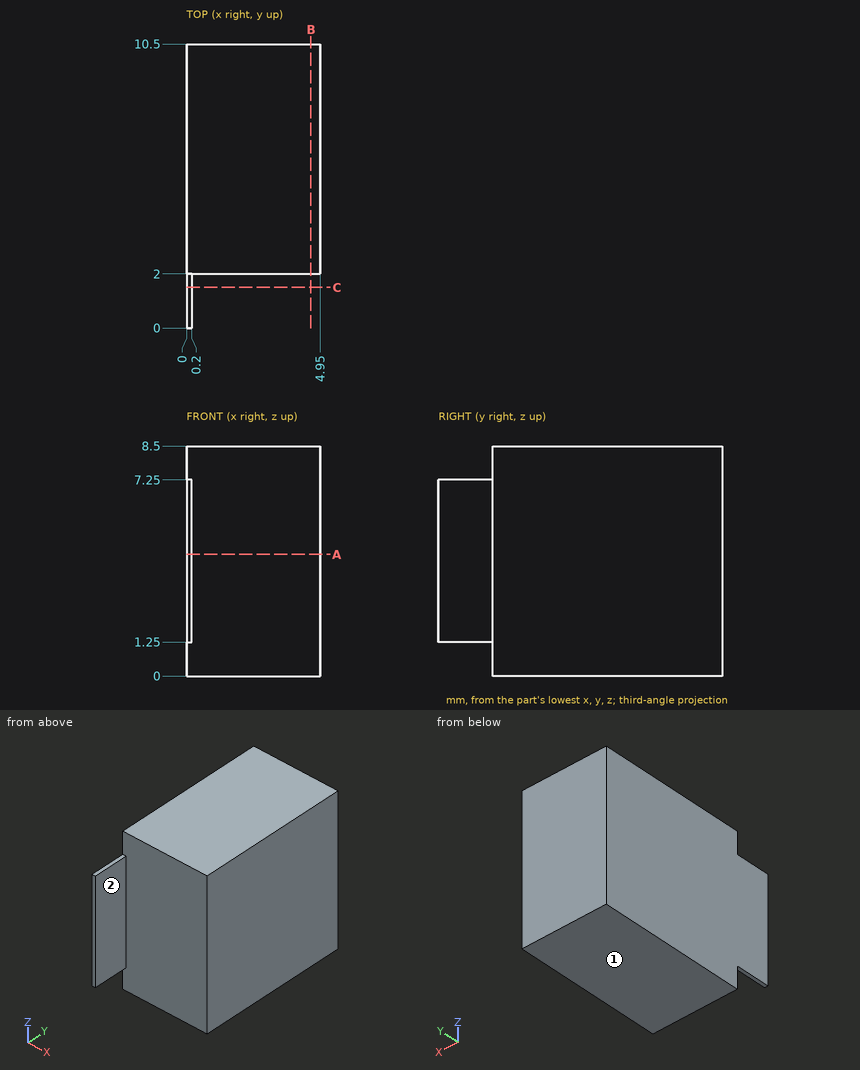
Part print with two shaded views. Sizes in mm from the minimum x, y, z corner. A direction names the side the tool comes from. Coordinates: 2 decimals unless noted, no trailing zeros. Write each loop counter-clockwise with the first axis right and the second up, starting at its lowest first coordinate (ties: lowest second). Pieces come first, ordered by that corner, then holes.
(1) 3-axis set-ups, long thin cutter, end or side, ignore diameter. For the marked faces 1 and 2: which of +Z, -Z, +X, -X, +Y, -Y reach the whole face in a straight line?
(2) Cut at A-A on z = 4.5. List the corners of the cut face in (x, y), and give its area (3 significant figures).
(3) Cut at C-C on y = 1.5. List the corners of the cut face in (x, z), and give its area (3 significant figures).
(4) Cut at B-B on x = 4.6. List the corners of the cut face in (y, z), and give its area (4 significant figures).
(5) Drill centre lines: line 1 (Y direction, x = 4.75, z = 5.5); line 2 (X direction, y = 1.5, z = 1.75). Where is each one in solid material? Low to high.
Working result:
1. face 1: -Z, +X, -X, +Y, -Y
1. face 2: +Z, -Z, +X, -Y
2. outline: (0, 0) - (0.2, 0) - (0.2, 2) - (4.95, 2) - (4.95, 10.5) - (0, 10.5) - close
2. area: 42.5 mm2
3. outline: (0, 1.25) - (0.2, 1.25) - (0.2, 7.25) - (0, 7.25) - close
3. area: 1.20 mm2
4. outline: (2, 0) - (10.5, 0) - (10.5, 8.5) - (2, 8.5) - close
4. area: 72.25 mm2
5. line 1: y = 2 to 10.5
5. line 2: x = 0 to 0.2
